Source: CAD feature listing. Evaluate the final solid. Frame: model axes, mm. A direction names the side the tool comes from. Coordinates: 2 decimals unless noted, no trailing zeros. Loops run counter-clockwise (first coordinate to the right, second up) from the corner with the lowest first, then second, coordinate; pieces in that order, holes last.
Item 1: Reachability of faces 1 (the cylindrical face through (12.4, -1.2, 1)), 2 (the flat face through (15, 0, -3)), 3 (the cylindrical face through (13.02, -13.57, -1.48)), 4 (the cylindrical face through (-13.02, 13.57, -1.48)), 5 (the flat face through (-20.56, -1.94, 0)) from +Z, -Z, +X, -X, +Y, -Y: full face, straight path, thin tool, end or side. Return the list, or none.
Item 2: Pin query (flat end, axial travel): pin 1 Ø2.5 at (x, y) = (0, -14) entering from -Z; pin 2 Ø22 at (x, y) = (6, 13.5) entering from -Z; pin 3 Ø2.5 at (x, y) = (-23, -2) entering from -Z; pin 4 Ø2 at (x, y) = (-14, 0.5) entering from +Z. Return the tip coordinate at first contact, or that it passes through.
Item 3: Section query C-C, the plane y = -14. Return the cut outline in (x, z), then the cut area to 3 significant figures.
Item 4: Line query: probe 1 along Y at (x, z) = (0, 1.25); probe 2 along Y at (x, z) = (21.5, -0.8); probe 3 along X at (y, z) = (13, -1.6). Output: solid intervals per line, ascending.
Item 5: Section query D-D, the plane x = -18. Return the cut outline in (y, z).
Item 6: Pull-direction query (X, two-part tool) for faces 6 (the flat face through (-15, 0, -3)), 7 (the flat face through (0, -19, 0)); classes: +X half, -X half, draft (parallel to the pull), parting line (faces both ways), or undercut.
Item 7: Section query B-B, the plane z = -1.25. Return the cut outline in (x, y).
Item 8: Section query A-A, the plane x = 0. Return the cut outline in (y, z), then the cut area to 3 significant figures.
```python
from build123d import *

# Parameters (mm, degrees)
SKETCH_R        = 27
SKETCH_R_2      = 10
PAD_DEPTH       = 2
SKETCH001_R     = 2
POCKET_DEPTH    = 2.001
SKETCH004_R     = 2
POCKET002_DEPTH = 2.001
SKETCH005_R     = 4.5
PAD001_DEPTH    = 3


with BuildPart() as part:
    # Sketch → Pad (new body)
    with BuildSketch(Plane.XY):
        Circle(SKETCH_R)
        Circle(SKETCH_R_2, mode=Mode.SUBTRACT)
    extrude(amount=PAD_DEPTH)

    # Sketch001 (on Face4 of Pad) → Pocket (cut, through all)
    with BuildSketch(Plane.XY.offset(2)):
        with Locations((0, 14)):
            Circle(SKETCH001_R)
        with Locations((14, 0)):
            Circle(SKETCH001_R)
        with Locations((0, -14)):
            Circle(SKETCH001_R)
        with Locations((-14, 0)):
            Circle(SKETCH001_R)
    extrude(amount=-POCKET_DEPTH, mode=Mode.SUBTRACT)

    # Sketch004 → Pocket002 (cut, through all)
    with BuildSketch(Plane.XY.offset(2)):
        with Locations((-21.5, 0)):
            Circle(SKETCH004_R)
        with Locations((21.5, 0)):
            Circle(SKETCH004_R)
    extrude(amount=-POCKET002_DEPTH, mode=Mode.SUBTRACT)

    # Sketch005 → Pad001 (join)
    with BuildSketch(Plane.XY):
        with BuildLine():
            ThreePointArc((21.75, 15.998047), (13.130278, 13.636266), (7.122093, 7.019672))
            ThreePointArc((7.122093, -7.019672), (10, 0), (7.122093, 7.019672))
            ThreePointArc((7.122093, -7.019672), (13.130278, -13.636266), (21.75, -15.998047))
            ThreePointArc((21.75, -15.998047), (27, 0), (21.75, 15.998047))
        make_face()
        with Locations((21.5, 0)):
            Circle(SKETCH005_R, mode=Mode.SUBTRACT)
        with BuildLine():
            ThreePointArc((-7.122093, 7.019672), (-10, 0), (-7.122093, -7.019672))
            ThreePointArc((-21.75, -15.998047), (-13.130278, -13.636266), (-7.122093, -7.019672))
            ThreePointArc((-21.75, 15.998047), (-27, 0), (-21.75, -15.998047))
            ThreePointArc((-7.122093, 7.019672), (-13.130278, 13.636266), (-21.75, 15.998047))
        make_face()
        with Locations((-21.5, 0)):
            Circle(SKETCH005_R, mode=Mode.SUBTRACT)
    extrude(amount=-PAD001_DEPTH)


solid = part.part
```
Verdict:
1. face 1: +Z
1. face 2: -Z, +X, -X, +Y, -Y
1. face 3: -Z, -Y
1. face 4: -Z, +Y
1. face 5: -Z
2. pin 1: passes through
2. pin 2: stops at z = -3
2. pin 3: stops at z = 0
2. pin 4: stops at z = 0
3. outline: (-23.09, -3) - (-13.75, -3) - (-13.75, 0) - (-2, 0) - (-2, 2) - (-23.09, 2) - close; (2, 0) - (13.75, 0) - (13.75, -3) - (23.09, -3) - (23.09, 2) - (2, 2) - close
3. area: 140 mm2
4. probe 1: y = -27 to -16, -12 to -10, 10 to 12, 16 to 27
4. probe 2: y = -16 to -4.5, 4.5 to 16
4. probe 3: x = -23.66 to -12.17, 12.17 to 23.66
5. outline: (-20.12, 0) - (-15.61, 0) - (-15.61, -3) - (-2.83, -3) - (-2.83, 0) - (2.83, 0) - (2.83, -3) - (15.61, -3) - (15.61, 0) - (20.12, 0) - (20.12, 2) - (-20.12, 2) - close
6. face 6: draft
6. face 7: undercut
7. outline: (-21.75, -16) arc R16 ccw to (-7.12, -7.02) arc R10 cw to (-7.12, 7.02) arc R16 ccw to (-21.75, 16) arc R27 ccw to start; (7.12, -7.02) arc R16 ccw to (21.75, -16) arc R27 ccw to (21.75, 16) arc R16 ccw to (7.12, 7.02) arc R10 cw to start; hole circle Ø9 at (-21.5, 0); hole circle Ø9 at (21.5, 0)
8. outline: (-27, 0) - (-16, 0) - (-16, 2) - (-27, 2) - close; (-12, 0) - (-10, 0) - (-10, 2) - (-12, 2) - close; (10, 0) - (12, 0) - (12, 2) - (10, 2) - close; (16, 0) - (27, 0) - (27, 2) - (16, 2) - close
8. area: 52.0 mm2
